Read the model definition and answer for the solid it produces. Units are mm, in the model's axes. A direction names the side the tool comes from. Give positions to 0.01 mm unless a question says otherwise; leave off trailing zeros. Write each loop counter-clockwise with the first axis right and the second up, starting at its lowest first coordinate (ties: lowest second). Pieces come first, ordered by that corner, then holes.
```python
from build123d import *

# Parameters (mm, degrees)
SKETCH4_R             = 1.651
SKETCH4_R_2           = 1.17475
BOSS_EXTRUDE1_DEPTH   = 1.5875
BOSS_EXTRUDE1_2_DEPTH = 1.5875
SKETCH5_R             = 1.14935
BOSS_EXTRUDE2_DEPTH   = 0.762


with BuildPart() as part:
    # Sketch4 → Boss-Extrude1 (new, symmetric)
    with BuildSketch(Plane.XY):
        with Locations((-3.175, 0)):
            Circle(SKETCH4_R)
        with Locations((-3.175, 0)):
            Circle(SKETCH4_R_2, mode=Mode.SUBTRACT)
    extrude(amount=BOSS_EXTRUDE1_DEPTH, both=True)


with BuildPart() as body_2:
    # Sketch4 → Boss-Extrude1 2 (new, symmetric)
    with BuildSketch(Plane.XY):
        with Locations((3.175, 0)):
            Circle(SKETCH4_R)
        with Locations((3.175, 0)):
            Circle(SKETCH4_R_2, mode=Mode.SUBTRACT)
    extrude(amount=BOSS_EXTRUDE1_2_DEPTH, both=True)


with BuildPart() as body_3:
    # Sketch5 → Boss-Extrude2 (new body)
    with BuildSketch(Plane.XY.offset(1.5875)):
        with BuildLine():
            ThreePointArc((-2.342877482, 2.879371452), (-6.1722, 0), (-2.342877482, -2.879371452))
            ThreePointArc((-2.342877482, -2.879371452), (0, -2.54762), (2.342877482, -2.879371452))
            ThreePointArc((2.342877482, -2.879371452), (6.1722, 0), (2.342877482, 2.879371452))
            ThreePointArc((2.342877482, 2.879371452), (0, 2.54762), (-2.342877482, 2.879371452))
        make_face()
        with Locations((-3.175, 0)):
            Circle(SKETCH5_R, mode=Mode.SUBTRACT)
        with Locations((3.175, 0)):
            Circle(SKETCH5_R, mode=Mode.SUBTRACT)
    extrude(amount=BOSS_EXTRUDE2_DEPTH)


with BuildPart() as body_4:
    # Mirror3: mirrored copy
    add(body_3.part.mirror(Plane.XY))

    # Combine2: union body 3, body 2, part
    add(body_3.part)
    add(body_2.part)
    add(part.part)


solid = body_4.part
```
Item 1: This flat-tipped pin is pushed along its axis until it touches: pin 1 Ø2.5 at (x, y) = (3.5, 0.5) entering from +Z. Where does it stop, or does it pass through?
Result set:
pin 1: stops at z = 2.35
Item 2: Section C-C (z = -1.4) is taken. Write down the section's boundary in (x, y) (1 decimal).
Result set:
outline: circle Ø3.3 at (-3.2, 0); circle Ø3.3 at (3.2, 0); hole circle Ø2.3 at (-3.2, 0); hole circle Ø2.3 at (3.2, 0)
Item 3: Determine the mould class of faces 1 (the cylindrical face through (2.263, -0.699, -1.963)), 2 (the cylindrical face through (-1.65, -0.63, 0.02)), 3 (the flat face through (0, 0, 1.588)) for opening direction Y: pulls with the +Y half, pulls with the -Y half, needs draft (parallel to the pull), parting line crosses it, or undercut.
Result set:
face 1: undercut
face 2: parting line crosses it
face 3: needs draft
Item 4: Section B-B (y = 0) is taken. Give the number of separate pieces and of enclosed holes in the cut face, and give its area (3 significant figures).
Result set:
separate pieces: 3
enclosed holes: 1
area: 17.9 mm2
Item 5: Section A-A (x = 0) is taken. Write down the section's boundary in (y, z), and give its area (3 significant figures).
Result set:
outline: (-2.55, -2.35) - (2.55, -2.35) - (2.55, -1.59) - (-2.55, -1.59) - close; (-2.55, 1.59) - (2.55, 1.59) - (2.55, 2.35) - (-2.55, 2.35) - close
area: 7.77 mm2
Item 6: Find the intervals of material crossed by line 1 along Z through (x, y) = (-3, -2.35); line 2 along Y through (x, z) = (-3.75, 0.35); line 3 along Y through (x, z) = (3, -1.1), in increasing order.
Result set:
line 1: z = -2.35 to -1.59, 1.59 to 2.35
line 2: y = -1.55 to -1.02, 1.02 to 1.55
line 3: y = -1.64 to -1.16, 1.16 to 1.64
Item 7: Section D-D (z = 1.95) is taken. Write down the section's boundary in (x, y) (1 decimal), and give its area (3 significant figures).
Result set:
outline: (-2.3, -2.9) arc R8.4 cw to (2.3, -2.9) arc R3 ccw (long way) to (2.3, 2.9) arc R8.4 cw to (-2.3, 2.9) arc R3 ccw (long way) to start; hole circle Ø2.3 at (-3.2, 0); hole circle Ø2.3 at (3.2, 0)
area: 54.7 mm2
Item 8: Which of the six approach directions +Z, -Z, +X, -X, +Y, -Y give full straight-line access (tool end or side, diameter ignored) to faces 4 (the cylindrical face through (2.263, -0.699, 1.963)), 5 (the flat face through (0, 0, -1.588))?
Result set:
face 4: +Z, -Z
face 5: none
